from build123d import *

# Parameters (mm, degrees)
SKETCH1_R           = 5.1
SKETCH1_R_2         = 3.5
BOSS_EXTRUDE2_DEPTH = 5
SKETCH2_R           = 2.5
CUT_EXTRUDE1_DEPTH  = 10
SKETCH3_W           = 322
SKETCH3_H           = 5
BOSS_EXTRUDE3_DEPTH = 106
SKETCH4_R           = 5.1
BOSS_EXTRUDE4_DEPTH = 5
SKETCH5_R           = 4
SKETCH5_W           = 30
SKETCH5_H           = 16
CUT_EXTRUDE2_DEPTH  = 10


with BuildPart() as part:
    # Sketch1 → Boss-Extrude2 (new body)
    with BuildSketch(Plane.XY):
        Polygon((-40, -40), (-10, -40), (-10, 10), (10, 10), (10, -40), (40, -40), (40, -120), (-40, -120), align=None)
        Circle(SKETCH1_R, mode=Mode.SUBTRACT)
        with Locations((0, -80)):
            Circle(SKETCH1_R_2, mode=Mode.SUBTRACT)
    extrude(amount=BOSS_EXTRUDE2_DEPTH)

    # Sketch2 → Cut-Extrude1 (cut)
    with BuildSketch(Plane.XY.offset(5)):
        with Locations((-23.57, -56.43)):
            Circle(SKETCH2_R)
        with Locations((23.57, -56.43)):
            Circle(SKETCH2_R)
        with Locations((-23.57, -103.57)):
            Circle(SKETCH2_R)
        with Locations((23.57, -103.57)):
            Circle(SKETCH2_R)
    extrude(amount=-CUT_EXTRUDE1_DEPTH, mode=Mode.SUBTRACT)

    # Sketch3 → Boss-Extrude3 (add)
    with BuildSketch(Plane.XY.offset(5)):
        with Locations((121, -117.5)):
            Rectangle(SKETCH3_W, SKETCH3_H)
    extrude(amount=BOSS_EXTRUDE3_DEPTH)

    # Sketch4 → Boss-Extrude4 (add)
    with BuildSketch(Plane.XY.offset(111)):
        Polygon((-40, -115), (-40, -120), (40, -120), (40, -115), (40, -40), (10, -40), (10, 10), (-10, 10), (-10, -40), (-40, -40), align=None)
        Circle(SKETCH4_R, mode=Mode.SUBTRACT)
    extrude(amount=BOSS_EXTRUDE4_DEPTH)

    # Sketch5 → Cut-Extrude2 (cut)
    with BuildSketch(Plane(origin=(0, -115, 0), x_dir=(1, 0, 0), z_dir=(0, 1, 0))):
        with Locations((0, -33.356338746)):
            Circle(SKETCH5_R)
        with Locations((0, -86.676260369)):
            Circle(SKETCH5_R)
        with Locations((230, -86.676260369)):
            Circle(SKETCH5_R)
        with Locations((230, -33.356338746)):
            Circle(SKETCH5_R)
        with Locations((267, -58)):
            Rectangle(SKETCH5_W, SKETCH5_H)
    extrude(amount=-CUT_EXTRUDE2_DEPTH, mode=Mode.SUBTRACT)


solid = part.part
Here's how the part is built. I have some questions about the finished solid (model axes, mm). A direction names the side the tool comes from. Coordinates: 2 decimals unless noted, no trailing zeros. Order: outer loops, then holes, each group sorted by start corner. A loop starts at its lowest first (then second) coordinate and runs counter-clockwise, first axis right, second up. Notation, with made-up numbers: (-20, 18) - (7, 18) arc R29 ccw to (7, 38) - close; hole circle Ø6 at (34.5, -12.5). An arc over 180 degrees is marked (long way). Use CSV: the item, a comma, the result in double quotes. Start each with the question number.
1. Suppose I cut it at C-C on y = -80. List the corners of the cut face in (x, z) for me, then the cut area to 3 significant figures.
2. I'm going to push flat-ended pins straight in: pin 1 (1.5 mm diameter, centred on x = 170.5, y = -116.5, fed in from -Z); pin 2 (4 mm diameter, centred on y = -98, z = 112.5, fed in from +X); pin 3 (2.5 mm diameter, centred on x = -28, z = 3, fed in from +Y); pin 4 (9 mm diameter, centred on x = 0, y = 0, fed in from +Z). Where does each tip first touch, or does it pass through?
3. Suppose I cut it at B-B on x = 0. List the corners of the cut face in (y, z) for me.
4. Please list where these lines run through material, in increasing order: line 1 (Y direction, x = 23.57, z = 3.5); line 2 (Y direction, x = 0, z = 1.85); line 3 (Z direction, x = -4.5, y = -27.5). Write a range as from..to.
5. Suppose I cut it at D-D on x = 230. List the corners of the cut face in (y, z) for me, then the cut area to 3 significant figures.
6. For faces 1 (the face through (119, -115, 57)), 2 (the face through (1, -69, 0)), 3 (the face through (-0.759, -83.417, 2.465)), which set-ups out of +Z, -Z, +X, -X, +Y, -Y let a thin tool reach every point of the face, with its end or its side?
7. Suppose I cut it at A-A on y = 0. List the corners of the cut face in (x, z) for me, then the cut area to 3 significant figures.
8. If we mould it in two halves opening along X, with no side actions, what happens to faces 4 (the face through (-1, -66, 111)), 5 (the face through (2.4, -4.5, 113.5)), 6 (the face through (-40, -115.4, 57.7))? For each: +X half, -X half, draft (parallel to the pull), parting line (faces both ways), or undercut.
Output:
1,outline,"(-40, 0) - (-3.5, 0) - (-3.5, 5) - (-40, 5) - close; (-40, 111) - (40, 111) - (40, 116) - (-40, 116) - close; (3.5, 0) - (40, 0) - (40, 5) - (3.5, 5) - close"
1,area,"765 mm2"
2,pin 1,"stops at z = 5"
2,pin 2,"stops at x = 40"
2,pin 3,"stops at y = -40"
2,pin 4,"passes through"
3,outline,"(-120, 0) - (-83.5, 0) - (-83.5, 5) - (-115, 5) - (-115, 29.36) - (-120, 29.36) - close; (-120, 37.36) - (-115, 37.36) - (-115, 82.68) - (-120, 82.68) - close; (-120, 90.68) - (-115, 90.68) - (-115, 111) - (-5.1, 111) - (-5.1, 116) - (-120, 116) - close; (-76.5, 0) - (-5.1, 0) - (-5.1, 5) - (-76.5, 5) - close; (5.1, 0) - (10, 0) - (10, 5) - (5.1, 5) - close; (5.1, 111) - (10, 111) - (10, 116) - (5.1, 116) - close"
4,line 1,"y = -120..-106.07, -101.07..-58.93, -53.93..-40"
4,line 2,"y = -120..-83.5, -76.5..-5.1, 5.1..10"
4,line 3,"z = 0..5, 111..116"
5,outline,"(-120, 5) - (-115, 5) - (-115, 29.36) - (-120, 29.36) - close; (-120, 37.36) - (-115, 37.36) - (-115, 82.68) - (-120, 82.68) - close; (-120, 90.68) - (-115, 90.68) - (-115, 111) - (-120, 111) - close"
5,area,"450 mm2"
6,face 1,"+X, -X, +Y"
6,face 2,"-Z, +X, -X, +Y, -Y"
6,face 3,"-Z"
7,outline,"(-10, 0) - (-5.1, 0) - (-5.1, 5) - (-10, 5) - close; (-10, 111) - (-5.1, 111) - (-5.1, 116) - (-10, 116) - close; (5.1, 0) - (10, 0) - (10, 5) - (5.1, 5) - close; (5.1, 111) - (10, 111) - (10, 116) - (5.1, 116) - close"
7,area,"98.0 mm2"
8,face 4,"draft"
8,face 5,"undercut"
8,face 6,"-X half"
